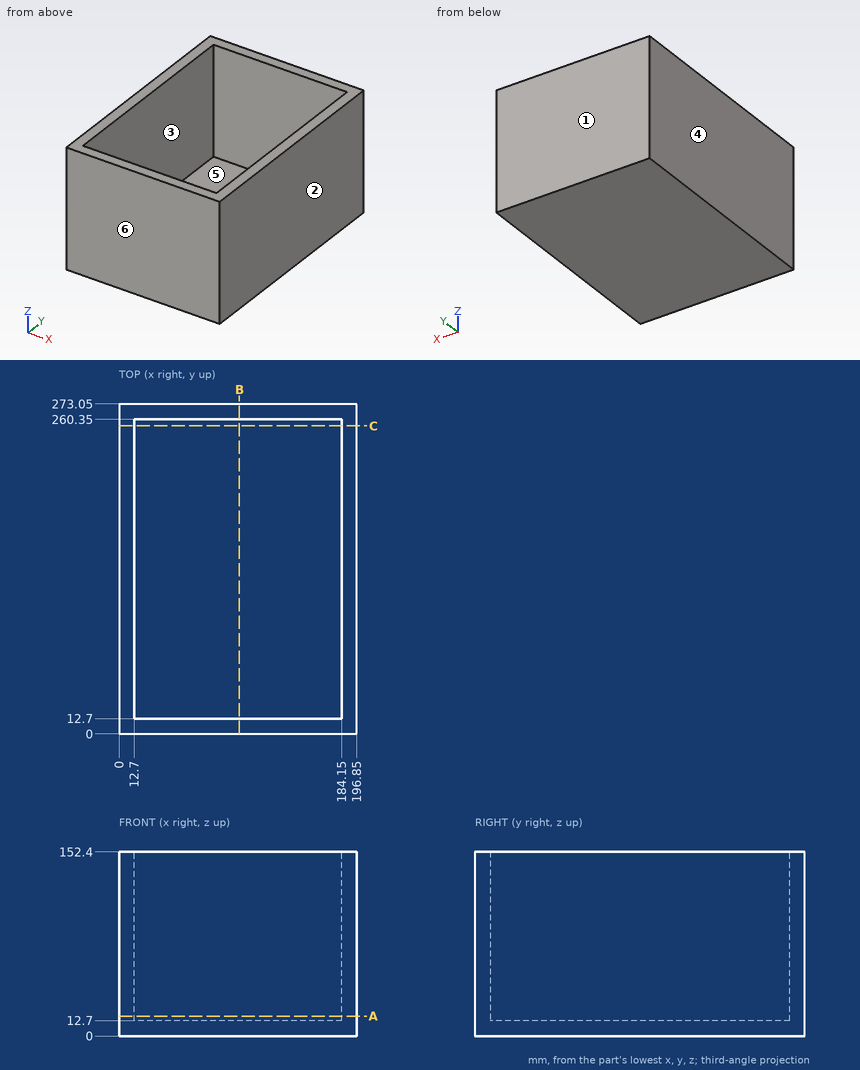
Geometry check sheet. Reference: drawing and pictorial views, mm from the part's lowest x, y, z. A direction names the side the tool comes from. Coordinates: 2 decimals unless noted, no trailing zeros. Loops run counter-clockwise (first coordinate to the right, second up) from the corner with the lowest first, then second, coordinate; pieces in that order, holes last.
1) Sectioned sample at B-B (x = 99.5). Record the boundary of the cut face in (y, z).
2) Release check for a two-part mould opening along X. For the marked faces 1, 2, 3 and 4 record: released by +X, released by -X, zero draft, split by the parting line, or undercut.
3) Sectioned sample at A-A (z = 16.5). Record the boundary of the cut face in (x, y), and give its area (3 significant figures).
4) Material ranges on probe 1 along X at (y, z) = (48, 77); probe 2 along Y at (x, z) = (163.5, 20.5); probe 3 along Z at (x, y) = (104.5, 114.5), recorded low to high.
5) Sectioned sample at C-C (y = 255). Record the boundary of the cut face in (x, z).
6) Gauge pin test, flat end, axial feed: pin 1 (3 mm diameter, centred on x = 164, y = 152.5, fed in from +Z). Record the tip position at first contact, or that the pin passes through.
7) Access from +Z, -Z, +X, -X, +Y, -Y to the whole of each face (thin tool, end or side, straight path). Record for the marked faces 5 and 6.
Check sheet entries:
1. outline: (0, 0) - (273.05, 0) - (273.05, 152.4) - (260.35, 152.4) - (260.35, 12.7) - (12.7, 12.7) - (12.7, 152.4) - (0, 152.4) - close
2. face 1: zero draft
2. face 2: released by +X
2. face 3: undercut
2. face 4: released by -X
3. outline: (0, 0) - (196.85, 0) - (196.85, 273.05) - (0, 273.05) - close; hole (12.7, 12.7) - (184.15, 12.7) - (184.15, 260.35) - (12.7, 260.35) - close
3. area: 11,300 mm2
4. probe 1: x = 0 to 12.7, 184.15 to 196.85
4. probe 2: y = 0 to 12.7, 260.35 to 273.05
4. probe 3: z = 0 to 12.7
5. outline: (0, 0) - (196.85, 0) - (196.85, 152.4) - (184.15, 152.4) - (184.15, 12.7) - (12.7, 12.7) - (12.7, 152.4) - (0, 152.4) - close
6. pin 1: stops at z = 12.7
7. face 5: +Z
7. face 6: +Z, -Z, +X, -X, -Y
